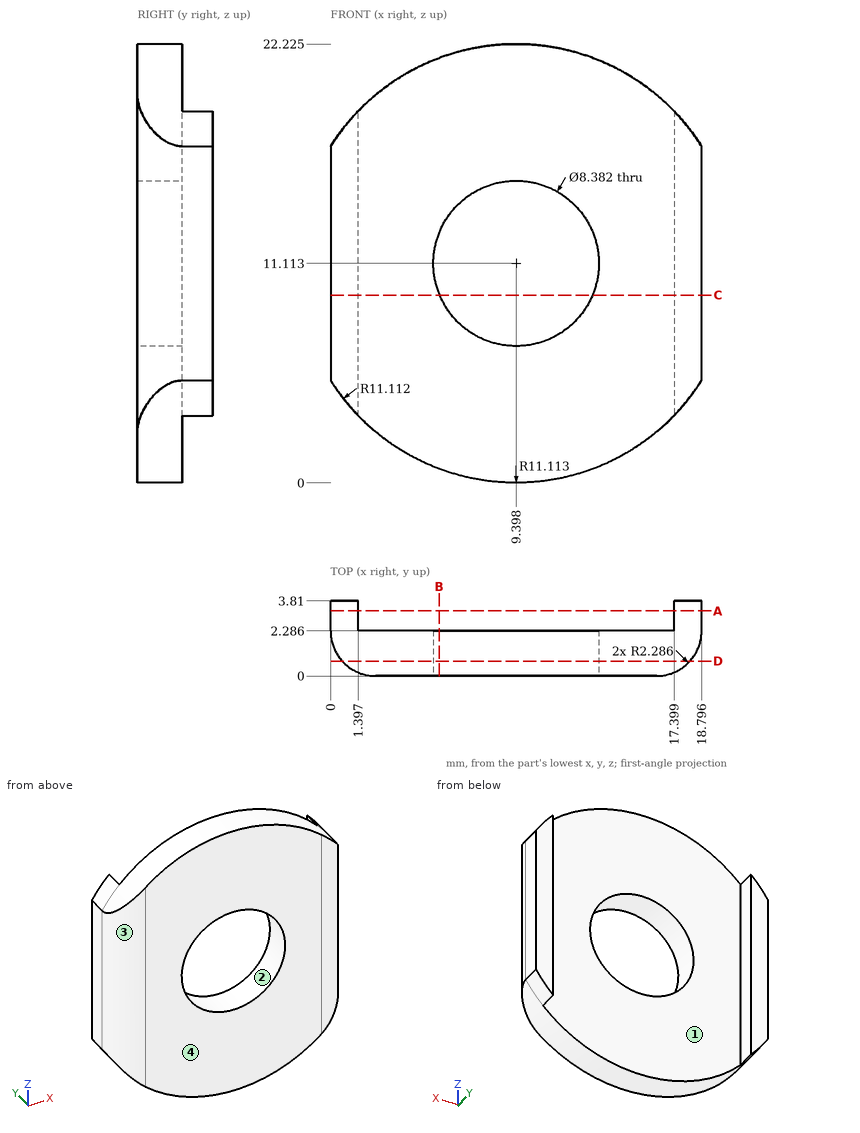
Can you work these out from the drawing? Everything is in mm from the part's minimum corner. Give positions to 0.01 mm unless a question says otherwise; leave off trailing zeros. Order: outer loops, then holes, each group sorted by start corner. A loop starts at its lowest first (then second) coordinate and runs counter-clockwise, first axis right, second up.
Item 1: If we mould it in two halves opening along X, with no side actions, what happens to the marked faces 1, 2, 3 and 4? For each: pulls with the +X half, pulls with the -X half, needs draft (parallel to the pull), parting line crosses it, or undercut.
Item 2: If we section it at A-A, the plane y = 3.3: Write out the boundary of the cut face in (x, z) (1 decimal).
Item 3: If we section it at D-D, the plane y = 0.75: Write out the boundary of the cut face in (x, z) (1 decimal).
Item 4: If we section it at B-B, the plane x = 5.5: Write out the boundary of the cut face in (y, z) (1 decimal).
Item 5: If we section it at C-C, the plane z = 9.5: Write out the boundary of the cut face in (x, y) (1 decimal).
Item 6: I need wall thicknesses on line 1 (X direction, y = 3.5, z = 12) (1 decimal); line 2 (Y direction, x = 2.25, z = 12.5) (1 decimal); line 3 (X direction, y = 0.4, z = 10.75) (1 decimal). Which ranges of each line are inside material? Lowest first, please.
Item 7: I'm going to push flat-ended pins straight in: pin 1 (1.5 mm diameter, centred on x = 12, y = 1.5, fed in from +Z); pin 2 (5 mm diameter, centred on x = 6, z = 8, fed in from +Y). Where does each tip first touch, or does it pass through?
Values:
1. face 1: undercut
1. face 2: undercut
1. face 3: pulls with the -X half
1. face 4: needs draft
2. outline: (0, 5.2) arc R11.1 ccw to (1.4, 3.4) - (1.4, 18.8) arc R11.1 ccw to (0, 17) - close; (17.4, 3.4) arc R11.1 ccw to (18.8, 5.2) - (18.8, 17) arc R11.1 ccw to (17.4, 18.8) - close
3. outline: (0.6, 4.3) arc R11.1 ccw to (18.2, 4.3) - (18.2, 17.9) arc R11.1 ccw to (0.6, 17.9) - close; hole circle Ø8.4 at (9.4, 11.1)
4. outline: (0, 0.7) - (2.3, 0.7) - (2.3, 9.6) - (0, 9.6) - close; (0, 12.7) - (2.3, 12.7) - (2.3, 21.5) - (0, 21.5) - close
5. outline: (0, 2.3) arc R2.3 ccw to (2.3, 0) - (5.5, 0) - (5.5, 2.3) - (1.4, 2.3) - (1.4, 3.8) - (0, 3.8) - close; (13.3, 0) - (16.5, 0) arc R2.3 ccw to (18.8, 2.3) - (18.8, 3.8) - (17.4, 3.8) - (17.4, 2.3) - (13.3, 2.3) - close
6. line 1: x = 0 to 1.4, 17.4 to 18.8
6. line 2: y = 0 to 2.3
6. line 3: x = 1 to 5.2, 13.6 to 17.8
7. pin 1: stops at z = 22.07
7. pin 2: stops at y = 2.29
